```python
from build123d import *

# Parameters (mm, degrees)
SKETCH1_W           = 42.3
SKETCH1_H           = 42.3
BOSS_EXTRUDE1_DEPTH = 34
SKETCH2_R           = 2.5
BOSS_EXTRUDE2_DEPTH = 24
SKETCH3_R           = 11
BOSS_EXTRUDE3_DEPTH = 2
SKETCH4_R           = 1.5
CUT_EXTRUDE1_DEPTH  = 4.5
CHAMFER1_SIZE       = 5
FILLET1_R           = 1


with BuildPart() as part:
    # Sketch1 → Boss-Extrude1 (new body)
    with BuildSketch(Plane(origin=(0, 0, 0), x_dir=(1, 0, 0), z_dir=(0, 1, 0))):
        Rectangle(SKETCH1_W, SKETCH1_H)
    extrude(amount=BOSS_EXTRUDE1_DEPTH)

    # Sketch2 → Boss-Extrude2 (add)
    with BuildSketch(Plane(origin=(0, 34, 0), x_dir=(1, 0, 0), z_dir=(0, 1, 0))):
        with Locations(Location((0, 0, 0), (0, 0, 90))):
            Circle(SKETCH2_R)
    extrude(amount=BOSS_EXTRUDE2_DEPTH)

    # Sketch3 → Boss-Extrude3 (add)
    with BuildSketch(Plane(origin=(0, 34, 0), x_dir=(1, 0, 0), z_dir=(0, 1, 0))):
        with Locations(Location((0, 0, 0), (0, 0, 90))):
            Circle(SKETCH3_R)
    extrude(amount=BOSS_EXTRUDE3_DEPTH)

    # Sketch4 → Cut-Extrude1 (cut)
    with BuildSketch(Plane(origin=(0, 34, 0), x_dir=(1, 0, 0), z_dir=(0, 1, 0))):
        with Locations(Location((-15.5, 15.5, 0), (0, 0, 270))):
            Circle(SKETCH4_R)
        with Locations(Location((15.5, 15.5, 0), (0, 0, 270))):
            Circle(SKETCH4_R)
        with Locations(Location((15.5, -15.5, 0), (0, 0, 270))):
            Circle(SKETCH4_R)
        with Locations(Location((-15.5, -15.5, 0), (0, 0, 270))):
            Circle(SKETCH4_R)
    extrude(amount=-CUT_EXTRUDE1_DEPTH, mode=Mode.SUBTRACT)

    # Chamfer1
    chamfer1_edges = [part.edges().sort_by_distance(p)[0] for p in [
        (21.15, 17, 21.15),
        (-21.15, 17, 21.15),
        (-21.15, 17, -21.15),
        (21.15, 17, -21.15),
    ]]
    chamfer(chamfer1_edges, length=CHAMFER1_SIZE)

    # Fillet1
    fillet1_edges = [part.edges().sort_by_distance(p)[0] for p in [
        (0, 58, 2.5),
    ]]
    fillet(fillet1_edges, radius=FILLET1_R)


solid = part.part
```
Input: part model. Units: mm. Frame: model coordinates. A direction names the side the tool comes from. Coordinates: 2 decimals unless noted, no trailing zeros. Loops run counter-clockwise (first coordinate to the right, second up) from the corner with the lowest first, then second, coordinate; pieces in that order, holes last. Notation, with made-up numbers: M -31.5,-25.75 L 22.5,-25.75 A7 ccw 22.5,-16.75 Z; hole C -39,52 d9. An arc over 180 degrees is marked long. One line per item, written item: value.
(1) Reachability of faces 1 (the flat face through (-15, 29.5, -16)), 2 (the flat face through (-18.6, 16.8, 18.7)) from +Z, -Z, +X, -X, +Y, -Y: full face, straight path, thin tool, end or side. Return the list, or none.
Filled in:
face 1: +Y
face 2: +Z, -X, +Y, -Y
(2) Pull-direction query (X, two-part tool) for faces 3 (the cylindrical face through (2.44, 46.35, 0.54)), 4 (the flat face through (0, 17, 21.15)), 5 (the cylindrical face through (15.57, 31.78, -17)); classes: +X half, -X half, draft (parallel to the pull), parting line (faces both ways), or undercut.
Filled in:
face 3: parting line
face 4: draft
face 5: undercut
(3) Section D-D (z = -18). Output: boundary loops of the cut face in (x, y).
Filled in:
outline: M -19.3,0 L 19.3,0 L 19.3,34 L -19.3,34 Z
(4) Section B-B (z = 0). Output: boundary loops of the cut face in (x, y), and give its area (3 significant figures).
Filled in:
outline: M -21.15,0 L 21.15,0 L 21.15,34 L 11,34 L 11,36 L 2.5,36 L 2.5,57 A1 ccw 1.5,58 L -1.5,58 A1 ccw -2.5,57 L -2.5,36 L -11,36 L -11,34 L -21.15,34 Z
area: 1,590 mm^2
(5) Line query: line 1 along X through (y, z) = (32.65, 15.5); line 2 along Z through (x, y) = (-15, 33). Output: solid intervals per line, ascending. Write a range as from..to.
Filled in:
line 1: -21.15..-17, -14..14, 17..21.15
line 2: -21.15..-16.91, -14.09..14.09, 16.91..21.15
(6) Section C-C (x = -8). Output: boundary loops of the cut face in (y, z), and give its area (3 significant figures).
Filled in:
outline: M 0,-21.15 L 34,-21.15 L 34,-7.55 L 36,-7.55 L 36,7.55 L 34,7.55 L 34,21.15 L 0,21.15 Z
area: 1,470 mm^2
(7) Section A-A (y = 14.5). Output: boundary loops of the cut face in (x, z).
Filled in:
outline: M -21.15,-16.15 L -16.15,-21.15 L 16.15,-21.15 L 21.15,-16.15 L 21.15,16.15 L 16.15,21.15 L -16.15,21.15 L -21.15,16.15 Z
(8) Pin query (flat end, axial travel): pin 1 (0.9 mm diameter, centred on x = -15, z = -15, fed in from +Y); pin 2 (4 mm diameter, centred on x = 15.5, z = -15.5, fed in from +Y); pin 3 (1 mm diameter, centred on x = 3.5, z = 10, fed in from +Y). Return the tip coordinate at first contact, or that it passes through.
Filled in:
pin 1: y = 29.5
pin 2: y = 34
pin 3: y = 36
